Input: dimensioned drawing with shaded views. Units: mm. Origin: part minimum x, y, z. Give positions to 0.01 mm unless a question says otherwise; leave off trailing zeros. Order: outer loops, then holes, each group sorted by start corner. A loop starts at its lowest first (then second) coordinate and runs counter-clockwise, first axis right, second up.
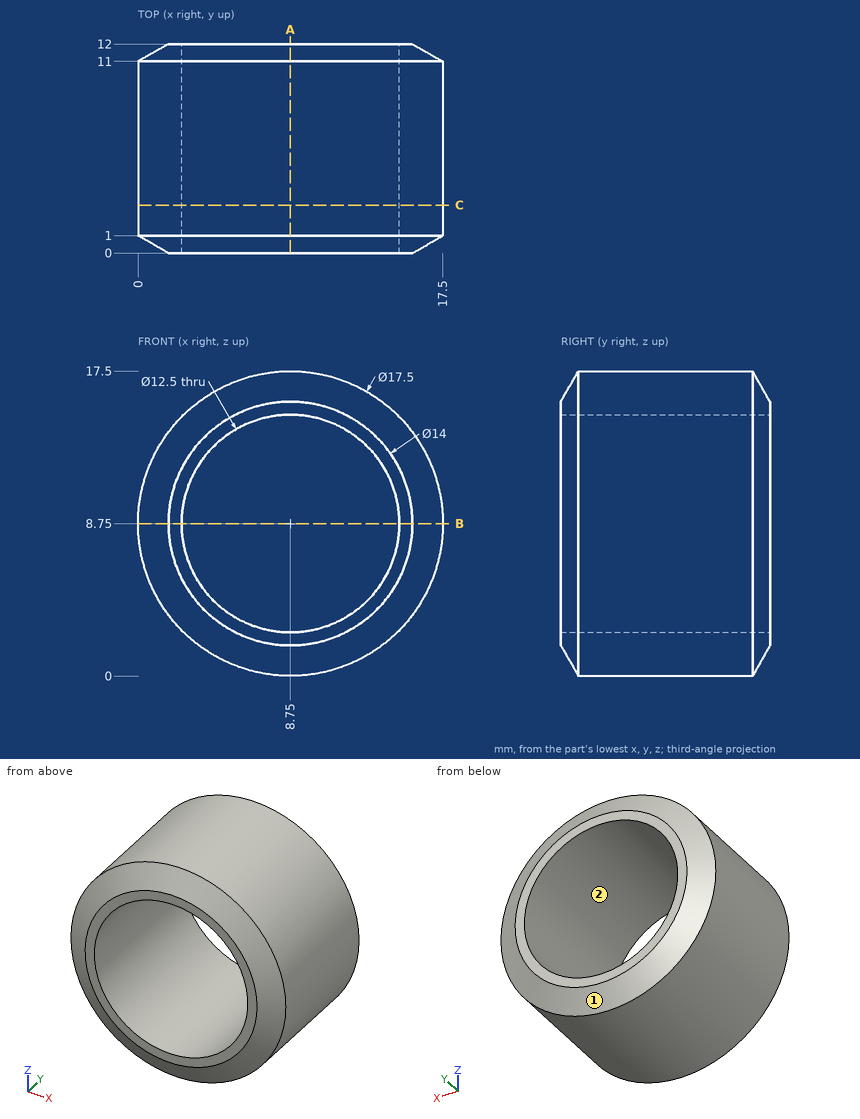
1) Line query: probe 1 along X at (y, z) = (5.5, 8.75); probe 2 along Z at (x, y) = (5, 2.25); probe 3 along Z at (x, y) = (6, 8). Output: solid intervals per line, ascending.
2) Cut plane B-B (z = 8.75). Return the cut outline in (x, y).
3) First-contact query: P1, Ø3, axis at x = 15.5, y = 8.5, coming from the +Z side; P2, Ø1, axis at y = 3, z = 15, coming from the +X side; P3, Ø3, axis at x = 6.5, y = 6, coming from the +Z side. Flat tips, straight axial feed; report the tip coordinate or a pass-through.
4) Pull-direction query (X, two-part tool) for the marked faces 1 and 2; classes: pulls with the +X half, pulls with the -X half, needs draft (parallel to the pull), parting line crosses it, or undercut.
5) Cut plane A-A (x = 8.75). Return the cut outline in (y, z), then the cut area to 3 significant figures.
6) Cut plane C-C (y = 2.75). Return the cut outline in (x, z).
Geometry says:
1. probe 1: x = 0 to 2.5, 15 to 17.5
1. probe 2: z = 0.84 to 3.75, 13.75 to 16.66
1. probe 3: z = 0.44 to 3.14, 14.36 to 17.06
2. outline: (0, 1) - (1.75, 0) - (2.5, 0) - (2.5, 12) - (1.75, 12) - (0, 11) - close; (15, 0) - (15.75, 0) - (17.5, 1) - (17.5, 11) - (15.75, 12) - (15, 12) - close
3. P1: stops at z = 15.75
3. P2: stops at x = 15.35
3. P3: stops at z = 17.47
4. face 1: parting line crosses it
4. face 2: undercut
5. outline: (0, 1.75) - (1, 0) - (11, 0) - (12, 1.75) - (12, 2.5) - (0, 2.5) - close; (0, 15) - (12, 15) - (12, 15.75) - (11, 17.5) - (1, 17.5) - (0, 15.75) - close
5. area: 56.5 mm2
6. outline: circle Ø17.5 at (8.75, 8.75); hole circle Ø12.5 at (8.75, 8.75)
